Can you work these out from the model? Positions are in its coordinate system, mm. A direction names the side the tool comes from. Round coordinates to 2 decimals unless told otherwise and drop trailing zeros. Write each loop counter-clockwise with the first axis right and the second up, starting at its lowest first coordinate (ties: lowest second). Pieces come first, ordered by that corner, then holes. Notation, with made-up numbers: M 60,46 L 76,46 A3 ccw 76,50 Z; hole C 69.5,-3 d5. An arc over 180 degrees is marked long. Answer as a JSON object with one key per item and string values. Group by question number.
1) On a 3-axis mill with a long thin cutter (end or side, diameter ignored), from which of +Z, -Z, +X, -X, +Y, -Y can I reach the whole of each face in a straight line? I mean faces 1 (the cylindrical face through (-1.18, 2.26, -14.86)), 2 (the cylindrical face through (23.846, 7.509, 2.465)). Say none if no direction works.
2) Suppose I cut it at D-D, the plane y = 9. Write out the boundary of the cut face in (x, z).
3) I'm going to push flat-ended pins straight in: pin 1 Ø1.5 at (y, z) = (15, -2.5) entering from -X; pin 2 Ø1.5 at (y, z) = (1.5, -4) entering from +X; pin 3 Ø2 at (x, y) = (-10, -14) entering from -Z; pin 4 Ø3 at (x, z) = (-2.5, -19) entering from -Y. Where does each tip first touch, or does it pass through?
4) Please list where these lines run through material, in increasing order: L1, parallel to Y at x = 0, z = 3.8; L2, parallel to Z at x = 10, y = -19.5; L3, parallel to Y at x = 0, z = -16.25. Write a range as [from, to].
5) If we mould it in two halves opening along X, with no side actions, what happens to faces 3 (the conical face through (-0.096, 0.432, -3.734)), 4 (the flat face through (0, 0, 5)), 5 (the cylindrical face through (-1.08, 4.88, -12.32))? For each: +X half, -X half, draft (parallel to the pull), parting line (faces both ways), or undercut.
6) Suppose I cut it at A-A, the plane y = -15. Write out the boundary of the cut face in (x, z).
7) Suppose I cut it at C-C, the plane z = -18. Write out the boundary of the cut face in (x, y), and give its area (3 significant figures).
from build123d import *

# Parameters (mm, degrees)
F0_R     = 25
F1_DEPTH = 5
F2_R     = 5
F3_DEPTH = 25
F5_D     = 5.1
F5_DEPTH = 20
F5_TIP   = 1.5321945785
F7_D     = 4
F7_DEPTH = 20
F7_TIP   = 1.2017212381


with BuildPart() as f1:
    # F0 (on Top) → F1 (new body)
    with BuildSketch(Plane.XY):
        Circle(F0_R)
    extrude(amount=F1_DEPTH)

    # F2 (on face) → F3 (join)
    with BuildSketch(Plane(origin=(0, 0, 0), x_dir=(1, 0, 0), z_dir=(0, 0, -1))):
        Circle(F2_R)
    extrude(amount=F3_DEPTH)

    # F5
    with Locations(Plane(origin=(0, 0, -25), x_dir=(1, 0, 0), z_dir=(0, 0, -1))):
        with Locations((0, 0)):
            Hole(F5_D / 2, depth=F5_DEPTH)
            with Locations((0, 0, -(F5_DEPTH + F5_TIP / 2))):  # 118° drill point
                Cone(0, F5_D / 2, F5_TIP, mode=Mode.SUBTRACT)

    # F7
    with Locations(Plane.XY.offset(5)):
        with Locations((0, 15), (-15, 0), (0, -15), (15, 0)):
            Hole(F7_D / 2, depth=F7_DEPTH)
            with Locations((0, 0, -(F7_DEPTH + F7_TIP / 2))):  # 118° drill point
                Cone(0, F7_D / 2, F7_TIP, mode=Mode.SUBTRACT)


solid = f1.part
Results:
{
 "1": {"face 1": "-Z", "face 2": "+Z, -Z"},
 "2": {"outline": "M -23.32,0 L 23.32,0 L 23.32,5 L -23.32,5 Z"},
 "3": {"pin 1": "through", "pin 2": "x = 4.94", "pin 3": "z = 0", "pin 4": "y = -4.9"},
 "4": {"L1": "[-25, -17], [-13, 13], [17, 25]", "L2": "[0, 5]", "L3": "[-5, -2.55], [2.55, 5]"},
 "5": {"face 3": "undercut", "face 4": "draft", "face 5": "parting line"},
 "6": {"outline": "M -20,0 L -2,0 L -2,5 L -20,5 Z; M 2,0 L 20,0 L 20,5 L 2,5 Z"},
 "7": {"outline": "C 0,0 d10; hole C 0,0 d5.1", "area": "58.1 mm^2"}
}
